Input: part model. Units: mm. Frame: model coordinates. Face numbers are marked on the shaded views. A direction names the side the tool comes from. Give positions to 0.01 mm unless a question says otherwise; leave off trailing zeros. Loops run counter-clockwise (first coordinate to the right, second up) from the corner with the lowest first, then second, coordinate; pieces in that order, holes last. Notation, with made-up numbers: (-12.75, -28.5) -> (12.25, -28.5) arc R24 cw to (12.25, -10.5) -> close; hole circle Ø5 at (37, -17.5). An arc over 180 degrees is marked (long way). Use CSV: the item, a comma, the result in double quotes.
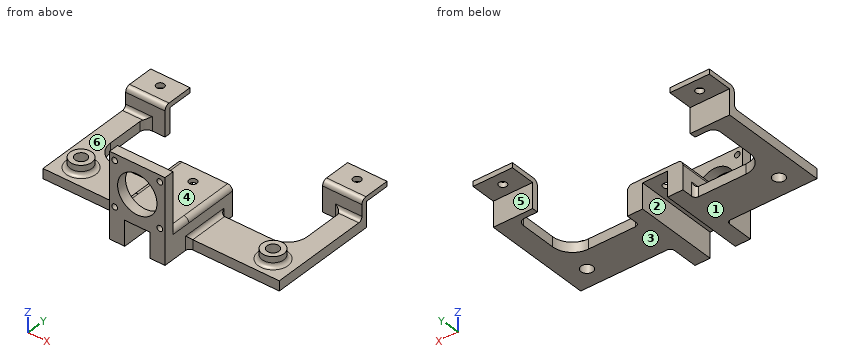
```python
from build123d import *

# Parameters (mm, degrees)
SKETCH19_R             = 6.05
BOSS_EXTRUDE12_DEPTH   = 10
BOSS_EXTRUDE12_2_DEPTH = 10
SKETCH20_R             = 11.05
SKETCH20_R_2           = 6.05
SKETCH20_W             = 40
SKETCH20_H             = 31.5
BOSS_EXTRUDE13_DEPTH   = 20.5
SKETCH21_W             = 25.5
SKETCH21_H             = 25.5
SKETCH21_W_2           = 10.5
SKETCH21_H_2           = 22.1
CUT_EXTRUDE11_DEPTH    = 269.086739694
CUT_EXTRUDE12_REACH    = 171.324
SKETCH22_R             = 4
BOSS_EXTRUDE14_DEPTH   = 55
FILLET6_R              = 5
BOSS_EXTRUDE16_DEPTH   = 20
SKETCH27_R             = 2.9
SKETCH27_R_2           = 20
BOSS_EXTRUDE15_DEPTH   = 10
FILLET10_R             = 4
SKETCH31_R             = 4
CUT_EXTRUDE13_DEPTH    = 10


with BuildPart() as part:
    # Sketch19 → Boss-Extrude12 (new body)
    with BuildSketch(Plane.XY):
        with BuildLine():
            Line((28.15, 20), (80, 20))
            ThreePointArc((80, 20), (94.142135624, 25.857864376), (100, 40))
            Line((100, 40), (100, 77))
            ThreePointArc((100, 77), (97.949747468, 81.949747468), (93, 84))
            Line((93, 84), (80, 84))
            Line((80, 84), (80, 115.5))
            Line((80, 115.5), (120, 115.5))
            Line((120, 115.5), (120, -20))
            Line((120, -20), (12.75, -20))
            Line((12.75, -20), (12.75, 20))
            Line((12.75, 20), (12.75, 35))
            Line((12.75, 35), (28.15, 35))
            Line((28.15, 35), (28.15, 20))
        make_face()
        with Locations((97.5, 0)):
            Circle(SKETCH19_R, mode=Mode.SUBTRACT)
    extrude(amount=BOSS_EXTRUDE12_DEPTH)



with BuildPart() as body_2:
    # Sketch19 → Boss-Extrude12 2 (new body)
    with BuildSketch(Plane.XY):
        with BuildLine():
            Line((-120, -20), (-12.75, -20))
            Line((-12.75, -20), (-12.75, 20))
            Line((-12.75, 20), (-12.75, 35))
            Line((-12.75, 35), (-28.15, 35))
            Line((-28.15, 35), (-28.15, 20))
            Line((-28.15, 20), (-80, 20))
            ThreePointArc((-80, 20), (-94.142135624, 25.857864376), (-100, 40))
            Line((-100, 40), (-100, 77))
            ThreePointArc((-100, 77), (-97.949747468, 81.949747468), (-93, 84))
            Line((-93, 84), (-80, 84))
            Line((-80, 84), (-80, 115.5))
            Line((-80, 115.5), (-120, 115.5))
            Line((-120, 115.5), (-120, -20))
        make_face()
        with Locations((-97.5, 0)):
            Circle(SKETCH19_R, mode=Mode.SUBTRACT)
    extrude(amount=BOSS_EXTRUDE12_2_DEPTH)


with BuildPart() as part_1:
    add(part.part)

    add(body_2.part)  # Boss-Extrude13 merges body 2
    # Sketch20 → Boss-Extrude13 (add)
    # profile 1 of 4: a face of its own
    with BuildSketch(Plane.XY.offset(10)):
        with Locations(Location((-97.5, 0, 0), (0, 0, 180))):
            Circle(SKETCH20_R)
        with Locations((-97.5, 0)):
            Circle(SKETCH20_R_2, mode=Mode.SUBTRACT)
    # profile 2 of 4: a face of its own
    with BuildSketch(Plane.XY.offset(10)):
        with Locations((97.5, 0)):
            Circle(SKETCH20_R)
        with Locations((97.5, 0)):
            Circle(SKETCH20_R_2, mode=Mode.SUBTRACT)
    # profile 3 of 4: a face of its own
    with BuildSketch(Plane.XY.offset(10)):
        with Locations((-100, 99.75)):
            Rectangle(SKETCH20_W, SKETCH20_H)
    # profile 4 of 4: a face of its own
    with BuildSketch(Plane.XY.offset(10)):
        with Locations((100, 99.75)):
            Rectangle(SKETCH20_W, SKETCH20_H)
    extrude(amount=BOSS_EXTRUDE13_DEPTH)

    # Sketch21 → Cut-Extrude11 (cut, through all)
    with BuildSketch(Plane(origin=(120, 0, 0), x_dir=(0, 0, -1), z_dir=(1, 0, 0))):
        with Locations((-12.75, 102.75)):
            Rectangle(SKETCH21_W, SKETCH21_H)
        with Locations((-25.25, 0)):
            Rectangle(SKETCH21_W_2, SKETCH21_H_2)
    extrude(amount=-CUT_EXTRUDE11_DEPTH, mode=Mode.SUBTRACT)

    # Sketch22 → Cut-Extrude12 (cut, up to next)
    with BuildSketch(Plane.XY.offset(30.5), mode=Mode.PRIVATE) as cut_extrude12_sk1:
        with Locations((-100, 102.75)):
            Circle(SKETCH22_R)
    cut_extrude12_tool1 = extrude(cut_extrude12_sk1.sketch, amount=-CUT_EXTRUDE12_REACH, mode=Mode.PRIVATE) & part_1.part
    # Sketch22 → Cut-Extrude12 (cut, up to next)
    with BuildSketch(Plane.XY.offset(30.5), mode=Mode.PRIVATE) as cut_extrude12_sk2:
        with Locations((100, 102.75)):
            Circle(SKETCH22_R)
    cut_extrude12_tool2 = extrude(cut_extrude12_sk2.sketch, amount=-CUT_EXTRUDE12_REACH, mode=Mode.PRIVATE) & part_1.part
    add(cut_extrude12_tool1.solids().sort_by_distance((-100, 102.75, 30.5))[0], mode=Mode.SUBTRACT)
    add(cut_extrude12_tool2.solids().sort_by_distance((100, 102.75, 30.5))[0], mode=Mode.SUBTRACT)

    # Sketch23 → Boss-Extrude14 (add)
    with BuildSketch(Plane.XZ.offset(20)):
        Polygon((-12.75, 10), (-28.15, 10), (-28.15, 29.5), (28.15, 29.5), (28.15, 10), (12.75, 10), (12.75, 25.5), (-12.75, 25.5), align=None)
    extrude(amount=-BOSS_EXTRUDE14_DEPTH)

    # Fillet6
    fillet6_edges = [part_1.edges().sort_by_distance(p)[0] for p in [
        (-28.15, 7.5, 29.5),
        (28.15, 7.5, 29.5),
        (100, 84, 30.5),
        (-100, 84, 30.5),
    ]]
    fillet(fillet6_edges, radius=FILLET6_R)

    # Sketch28 → Boss-Extrude16 (add)
    with BuildSketch(Plane.XZ.offset(20)):
        with BuildLine():
            Line((-28.15, 0), (-28.15, 24.5))
            ThreePointArc((-28.15, 24.5), (-26.685533906, 28.035533906), (-23.15, 29.5))
            Line((-23.15, 29.5), (23.15, 29.5))
            ThreePointArc((23.15, 29.5), (26.685533906, 28.035533906), (28.15, 24.5))
            Line((28.15, 24.5), (28.15, 0))
            Line((28.15, 0), (12.75, 0))
            Line((12.75, 0), (12.75, 25.5))
            Line((12.75, 25.5), (-12.75, 25.5))
            Line((-12.75, 25.5), (-12.75, 0))
            Line((-12.75, 0), (-28.15, 0))
        make_face()
    extrude(amount=BOSS_EXTRUDE16_DEPTH)

    # Sketch27 → Boss-Extrude15 (add)
    with BuildSketch(Plane(origin=(0, -40, 0), x_dir=(1, 0, 0), z_dir=(0, 1, 0))):
        Polygon((-12.75, 0), (-12.75, -25.5), (12.75, -25.5), (12.75, 0), (28.15, 0), (28.15, -85.9), (-28.15, -85.9), (-28.15, 0), align=None)
        with Locations(Location((-22.95, -79.3, 0), (0, 0, 180))):
            Circle(SKETCH27_R, mode=Mode.SUBTRACT)
        with Locations(Location((22.95, -79.3, 0), (0, 0, 180))):
            Circle(SKETCH27_R, mode=Mode.SUBTRACT)
        with Locations(Location((22.95, -33.8, 0), (0, 0, 180))):
            Circle(SKETCH27_R, mode=Mode.SUBTRACT)
        with Locations(Location((-22.95, -33.8, 0), (0, 0, 180))):
            Circle(SKETCH27_R, mode=Mode.SUBTRACT)
        with Locations(Location((0, -56.55, 0), (0, 0, 180))):
            Circle(SKETCH27_R_2, mode=Mode.SUBTRACT)
    extrude(amount=-BOSS_EXTRUDE15_DEPTH)

    # Fillet10
    fillet10_edges = [part_1.edges().sort_by_distance(p)[0] for p in [
        (-28.15, 0, 10),
        (28.15, 0, 10),
        (106.5, 84, 10),
        (28.15, 20, 5),
        (86.45, 0, 10),
        (-28.15, 20, 5),
        (-28.15, -20, 5),
        (28.15, -20, 5),
        (-86.45, 0, 10),
        (-106.5, 84, 10),
    ]]
    fillet(fillet10_edges, radius=FILLET10_R)

    # Sketch31 → Cut-Extrude13 (cut)
    with BuildSketch(Plane.XY.offset(29.5)):
        with Locations((0, 20)):
            Circle(SKETCH31_R)
    extrude(amount=-CUT_EXTRUDE13_DEPTH, mode=Mode.SUBTRACT)


solid = part_1.part
```
1) Section query B-B (y = 43). Return loops of the section in (x, z), then the cut area to 3 significant figures.
From the geometry:
outline,"(-120, 0) -> (-100, 0) -> (-100, 10) -> (-120, 10) -> close; (100, 0) -> (120, 0) -> (120, 10) -> (100, 10) -> close"
area,"400 mm^2"
2) Contact query for flat-ended pins moving along their axis: pin 1 (7.5 mm diameter, centred on x = -97, z = 12.5, fed in from +Y); pin 2 (8 mm diameter, centred on x = -95, y = 2.5, fed in from +Z); pin 3 (1 mm diameter, centred on y = -28, z = 24, fed in from +X); pin 4 (20.5 mm diameter, centred on y = -20.5, z = 8, fed in from +X). Output: stop coordinate, or through.
From the geometry:
pin 1,"stops at y = 90"
pin 2,"stops at z = 20"
pin 3,"stops at x = 28.15"
pin 4,"stops at x = 120"
3) Section query D-D (x = -9). Return loops of the section in (y, z).
From the geometry:
outline,"(-50, 25.5) -> (35, 25.5) -> (35, 29.5) -> (-40, 29.5) -> (-40, 38.69) -> (-50, 38.69) -> close; (-50, 74.41) -> (-40, 74.41) -> (-40, 85.9) -> (-50, 85.9) -> close"
4) Mould query, pull axis X, two halves, no side actions, for the marked faces 1 and 2. Classes: pulls with the +X half, pulls with the -X half, needs draft (parallel to the pull), parting line crosses it, or undercut.
From the geometry:
face 1,"needs draft"
face 2,"undercut"
5) Ray query, line 1 (Z direction, x = 22.95, y = -43.5); line 2 (Y direction, x = 97.5, z = 8.5); line 3 (X direction, y = 10, z = 24). Return the intervals inside material, ascending.
From the geometry:
line 1,"z = 0 to 30.9, 36.7 to 76.4, 82.2 to 85.9"
line 2,"y = -20 to -6.05, 6.05 to 30.32, 82.36 to 90"
line 3,"x = -28.15 to -12.75, 12.75 to 28.15"
6) Section query C-C (y = 102.75). Return loops of the section in (x, z).
From the geometry:
outline,"(-120, 25.5) -> (-104, 25.5) -> (-104, 30.5) -> (-120, 30.5) -> close; (-96, 25.5) -> (-80, 25.5) -> (-80, 30.5) -> (-96, 30.5) -> close; (80, 25.5) -> (96, 25.5) -> (96, 30.5) -> (80, 30.5) -> close; (104, 25.5) -> (120, 25.5) -> (120, 30.5) -> (104, 30.5) -> close"
7) Reachability of the marked faces 3, 4, 5 and 6 from +Z, -Z, +X, -X, +Y, -Y: full face, straight path, thin tool, end or side. Return the list, or none.
From the geometry:
face 3,"-Z, +X, -X, +Y, -Y"
face 4,"+Z, +X, -X, +Y"
face 5,"-Z, +X, -X, +Y"
face 6,"+Z"
8) Section query A-A (z = 33.8). Return loops of the section in (x, y), then the cut area to 3 significant figures.
From the geometry:
outline,"(-28.15, -50) -> (-25.85, -50) -> (-25.85, -40) -> (-28.15, -40) -> close; (-20.05, -50) -> (20.05, -50) -> (20.05, -40) -> (-20.05, -40) -> close; (25.85, -50) -> (28.15, -50) -> (28.15, -40) -> (25.85, -40) -> close"
area,"447 mm^2"
